The model under review builds one solid part; all positions refer to its coordinate system, in mm. A direction names the side the tool comes from. Round coordinates to 2 decimals unless told otherwise and drop trailing zeros. Loops run counter-clockwise (first coordinate to the right, second up) from the corner with the lowest first, then second, coordinate; pieces in that order, holes last. Notation, with made-up numbers: (28.5, 72) -> (71.5, 72) arc R11 ccw to (71.5, 78) -> close; hole circle Ø8 at (40, 53). An arc over 180 degrees is marked (long way). Write each question's results on one line, items separated by ' | '. Start each with the question number.
Item 1: We need section C-C (x = -1.25). Give the boundary of the cut face in (y, z), and give its area (3 significant figures).
Item 2: We need section D-D (y = -3). Give the boundary of the cut face in (x, z), and give its area (3 significant figures).
Item 3: Tool access review of faces 1 (the flat face through (3, -3.5, 34)), 2 (the cylindrical face through (2.64, 3.04, 44.4)), 3 (the flat face through (-6, 0, 27)): name each direction out of +Z, -Z, +X, -X, +Y, -Y from which nothing blocks a thin tool from reaching the whole face with its end or side.
Item 4: Mouldability with a two-part tool opening along X and no side actions: class faces 4 (the flat face through (0, -1, 8)), 5 (the cylindrical face through (-2.64, 3.04, 23.6)), 6 (the cylindrical face through (3.04, -2.6, 2.36)) as pulls with the +X half, pulls with the -X half, needs draft (parallel to the pull), parting line crosses it, or undercut.
Item 5: For L1, parallel to Z at x = 3.75, y = 0; L2, parallel to Z at x = -4.3, y = 0; L3, parallel to Z at x = 3.25, y = 2.5, list the stretches that pass through material, from the lowest coordinate up. Write a range as from..to.
Item 6: We need section A-A (x = 5). Give the boundary of the cut face in (y, z), and give its area (3 significant figures).
Item 7: Clearance check with a flat-ended pin moving along its axis: pin 1 Ø5 at (x, z) = (0, 48) entering from +Y. State where the tip first meets the part, or that it passes through.
Item 8: We need section B-B (z = 34). Give the boundary of the cut face in (x, y), and give its area (3 significant figures).
from build123d import *

# Parameters (mm, degrees)
SKETCH1_W           = 12
SKETCH1_H           = 12
BOSS_EXTRUDE1_DEPTH = 54
SKETCH2_R           = 2
CUT_EXTRUDE1_DEPTH  = 14
SKETCH3_R           = 2
CUT_EXTRUDE2_DEPTH  = 14
CUT_EXTRUDE3_DEPTH  = 6
CUT_EXTRUDE4_DEPTH  = 6


with BuildPart() as part:
    # Sketch1 → Boss-Extrude1 (new body)
    with BuildSketch(Plane.XY):
        Rectangle(SKETCH1_W, SKETCH1_H)
    extrude(amount=BOSS_EXTRUDE1_DEPTH)

    # Sketch2 → Cut-Extrude1 (cut)
    with BuildSketch(Plane(origin=(0, 6, 0), x_dir=(1, 0, 0), z_dir=(0, 1, 0))):
        with Locations(Location((0, -20, 0), (0, 0, 180))):
            Circle(SKETCH2_R)
        with Locations(Location((0, -48, 0), (0, 0, 180))):
            Circle(SKETCH2_R)
    extrude(amount=-CUT_EXTRUDE1_DEPTH, mode=Mode.SUBTRACT)

    # Sketch3 → Cut-Extrude2 (cut)
    with BuildSketch(Plane.ZY.offset(6)):
        with Locations(Location((34, 0, 0), (0, 0, 270))):
            Circle(SKETCH3_R)
        with Locations(Location((6, 0, 0), (0, 0, 270))):
            Circle(SKETCH3_R)
    extrude(amount=-CUT_EXTRUDE2_DEPTH, mode=Mode.SUBTRACT)

    # Sketch4 → Cut-Extrude3 (cut)
    with BuildSketch(Plane(origin=(6, 0, 0), x_dir=(0, 0, -1), z_dir=(1, 0, 0))):
        with BuildLine():
            Line((-4.5, -3.5), (-7.5, -3.5))
            ThreePointArc((-7.5, -3.5), (-9.621320344, -2.621320344), (-10.5, -0.5))
            Line((-10.5, -0.5), (-10.5, 0.5))
            ThreePointArc((-10.5, 0.5), (-9.621320344, 2.621320344), (-7.5, 3.5))
            Line((-7.5, 3.5), (-4.5, 3.5))
            ThreePointArc((-4.5, 3.5), (-2.378679656, 2.621320344), (-1.5, 0.5))
            Line((-1.5, 0.5), (-1.5, -0.5))
            ThreePointArc((-1.5, -0.5), (-2.378679656, -2.621320344), (-4.5, -3.5))
        make_face()
        with BuildLine():
            Line((-38.5, -0.5), (-38.5, 0.5))
            ThreePointArc((-38.5, 0.5), (-37.621320344, 2.621320344), (-35.5, 3.5))
            Line((-35.5, 3.5), (-32.5, 3.5))
            ThreePointArc((-32.5, 3.5), (-30.378679656, 2.621320344), (-29.5, 0.5))
            Line((-29.5, 0.5), (-29.5, -0.5))
            ThreePointArc((-29.5, -0.5), (-30.378679656, -2.621320344), (-32.5, -3.5))
            Line((-32.5, -3.5), (-35.5, -3.5))
            ThreePointArc((-35.5, -3.5), (-37.621320344, -2.621320344), (-38.5, -0.5))
        make_face()
    extrude(amount=-CUT_EXTRUDE3_DEPTH, mode=Mode.SUBTRACT)

    # Sketch5 → Cut-Extrude4 (cut)
    with BuildSketch(Plane(origin=(0, 6, 0), x_dir=(1, 0, 0), z_dir=(0, 1, 0))):
        with BuildLine():
            Line((-0.5, -52.5), (0.5, -52.5))
            ThreePointArc((0.5, -52.5), (2.621320344, -51.621320344), (3.5, -49.5))
            Line((3.5, -49.5), (3.5, -46.5))
            ThreePointArc((3.5, -46.5), (2.621320344, -44.378679656), (0.5, -43.5))
            Line((0.5, -43.5), (-0.5, -43.5))
            ThreePointArc((-0.5, -43.5), (-2.621320344, -44.378679656), (-3.5, -46.5))
            Line((-3.5, -46.5), (-3.5, -49.5))
            ThreePointArc((-3.5, -49.5), (-2.621320344, -51.621320344), (-0.5, -52.5))
        make_face()
        with BuildLine():
            Line((-0.5, -24.5), (0.5, -24.5))
            ThreePointArc((0.5, -24.5), (2.621320344, -23.621320344), (3.5, -21.5))
            Line((3.5, -21.5), (3.5, -18.5))
            ThreePointArc((3.5, -18.5), (2.621320344, -16.378679656), (0.5, -15.5))
            Line((0.5, -15.5), (-0.5, -15.5))
            ThreePointArc((-0.5, -15.5), (-2.621320344, -16.378679656), (-3.5, -18.5))
            Line((-3.5, -18.5), (-3.5, -21.5))
            ThreePointArc((-3.5, -21.5), (-2.621320344, -23.621320344), (-0.5, -24.5))
        make_face()
    extrude(amount=-CUT_EXTRUDE4_DEPTH, mode=Mode.SUBTRACT)


solid = part.part
Here are the results:
1) outline: (-6, 0) -> (6, 0) -> (6, 15.6) -> (0, 15.6) -> (0, 18.44) -> (-6, 18.44) -> close; (-6, 21.56) -> (0, 21.56) -> (0, 24.4) -> (6, 24.4) -> (6, 43.6) -> (0, 43.6) -> (0, 46.44) -> (-6, 46.44) -> close; (-6, 49.56) -> (0, 49.56) -> (0, 52.4) -> (6, 52.4) -> (6, 54) -> (-6, 54) -> close; hole circle Ø4 at (0, 6); hole circle Ø4 at (0, 34) | area: 480 mm2
2) outline: (-6, 0) -> (6, 0) -> (6, 2.84) -> (0, 2.84) -> (0, 9.16) -> (6, 9.16) -> (6, 30.84) -> (0, 30.84) -> (0, 37.16) -> (6, 37.16) -> (6, 54) -> (-6, 54) -> close; hole circle Ø4 at (0, 20); hole circle Ø4 at (0, 48) | area: 547 mm2
3) face 1: +X | face 2: +Y | face 3: +Z, -Z, -X, +Y, -Y
4) face 4: pulls with the +X half | face 5: undercut | face 6: needs draft
5) L1: z = 0..1.5, 10.5..29.5, 38.5..54 | L2: z = 0..4, 8..32, 36..54 | L3: z = 0..2.26, 9.74..17.3, 22.7..30.26, 37.74..45.3, 50.7..54
6) outline: (-6, 0) -> (6, 0) -> (6, 54) -> (-6, 54) -> close; hole (-3.5, 4.5) arc R3 ccw to (-0.5, 1.5) -> (0.5, 1.5) arc R3 ccw to (3.5, 4.5) -> (3.5, 7.5) arc R3 ccw to (0.5, 10.5) -> (-0.5, 10.5) arc R3 ccw to (-3.5, 7.5) -> close; hole (-3.5, 32.5) arc R3 ccw to (-0.5, 29.5) -> (0.5, 29.5) arc R3 ccw to (3.5, 32.5) -> (3.5, 35.5) arc R3 ccw to (0.5, 38.5) -> (-0.5, 38.5) arc R3 ccw to (-3.5, 35.5) -> close | area: 537 mm2
7) pin 1: stops at y = 0
8) outline: (-6, -6) -> (6, -6) -> (6, -3.5) -> (0, -3.5) -> (0, -2) -> (-6, -2) -> close; (-6, 2) -> (0, 2) -> (0, 3.5) -> (6, 3.5) -> (6, 6) -> (-6, 6) -> close | area: 78.0 mm2
